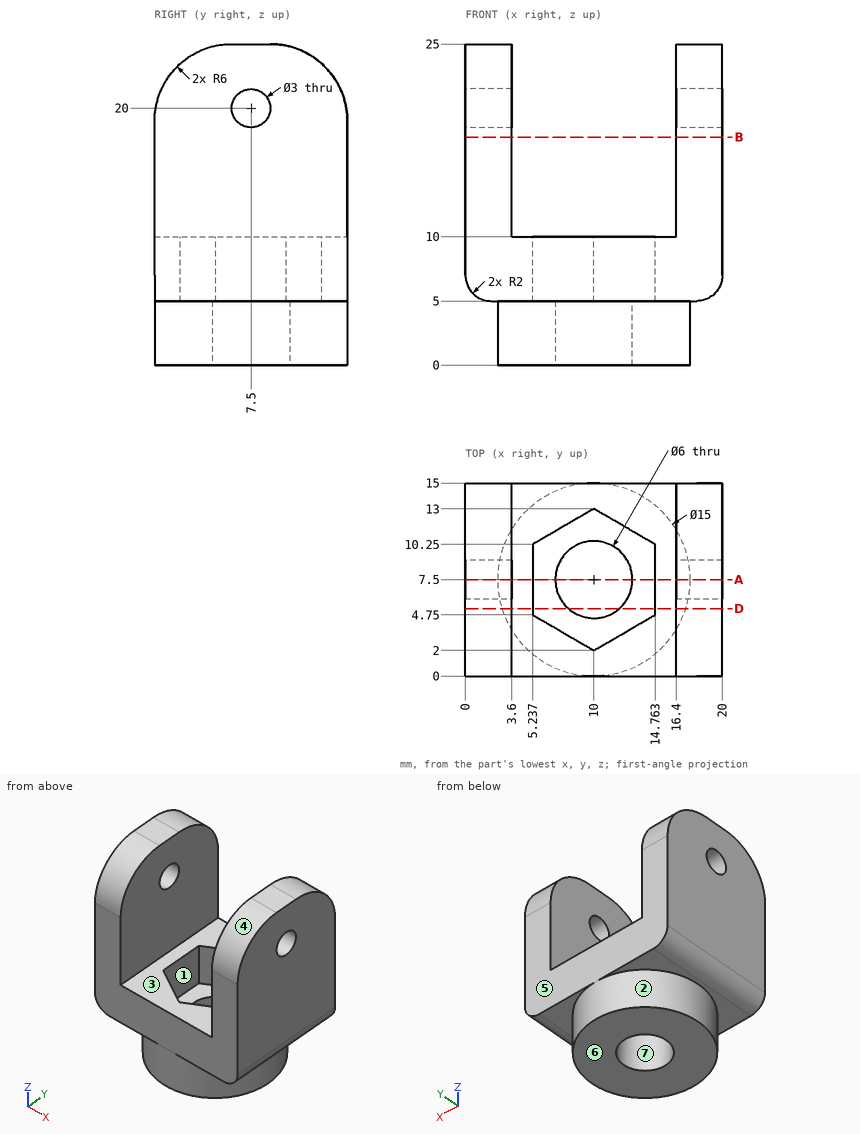
The drawing under review shows one solid part. Ordinate dimensions are in mm from its lowest x, y, z. A direction names the side the tool comes from. Round coordinates to 2 decimals unless told otherwise and drop trailing zeros. Write each loop counter-clockwise with the first axis right and the second up, starting at its lowest first coordinate (ties: lowest second). Pieces come first, ordered by that corner, then holes. Notation, with made-up numbers: (29.5, -31) -> (64.5, -31) arc R13 cw to (64.5, -14) -> close; hole circle Ø4 at (18.25, -29). An arc over 180 degrees is marked (long way). One line per question, with ' | ' between items.
(1) Wall thickness on line 1 (X direction, y = 14, z = 19.5); line 2 (X direction, y = 8.25, z = 9.5); line 3 (Z direction, x = 17.75, y = 7.5): over which ranges is each line inside the solid? List them lowest first. Write a range as [from, to].
Result sheet:
line 1: [0, 3.6], [16.4, 20] | line 2: [0, 5.24], [14.76, 20] | line 3: [5, 18.5], [21.5, 25]
(2) Take a section at D-D, the plane y = 5.25. State the section outline as (x, z) points.
Result sheet:
outline: (0, 7) arc R2 ccw to (2, 5) -> (2.85, 5) -> (2.85, 0) -> (8.02, 0) -> (8.02, 5) -> (5.24, 5) -> (5.24, 10) -> (3.6, 10) -> (3.6, 24.95) -> (0, 24.95) -> close; (11.98, 0) -> (17.15, 0) -> (17.15, 5) -> (18, 5) arc R2 ccw to (20, 7) -> (20, 24.95) -> (16.4, 24.95) -> (16.4, 10) -> (14.76, 10) -> (14.76, 5) -> (11.98, 5) -> close
(3) Take a section at B-B, the plane z = 17.75. State the section outline as (x, y) points, and give its area (3 significant figures).
Result sheet:
outline: (0, 0) -> (3.6, 0) -> (3.6, 15) -> (0, 15) -> close; (16.4, 0) -> (20, 0) -> (20, 15) -> (16.4, 15) -> close | area: 108 mm2
(4) Machinability: for the marked faces 1, 2 and 3, which of the approach directions +Z, -Z, +X, -X, +Y, -Y give a long, thin tool a straight path to every point of the face, cutting with its end or side? Answer none if there is none.
Result sheet:
face 1: +Z | face 2: -Z | face 3: +Z, +Y, -Y
(5) Draft analysis for pull direction Y (two halves, no side actions). For the marked faces 4, 5, 6 and 7, state which applies: released by +Y, released by -Y, zero draft, split by the parting line, or undercut.
Result sheet:
face 4: released by -Y | face 5: released by +Y | face 6: zero draft | face 7: undercut
(6) Take a section at A-A, the plane y = 7.5. State how many separate pieces and enclosed holes the cut face has, and give its area (3 significant figures).
Result sheet:
separate pieces: 4 | enclosed holes: 0 | area: 182 mm2
(7) Insertion check: P1, Ø5, axis at x = 10, y = 5, coming from the +Z side. The pin has a flat end and moves straight along its axis. Give the tip position at first contact, or say it passes through.
Result sheet:
P1: z = 5
